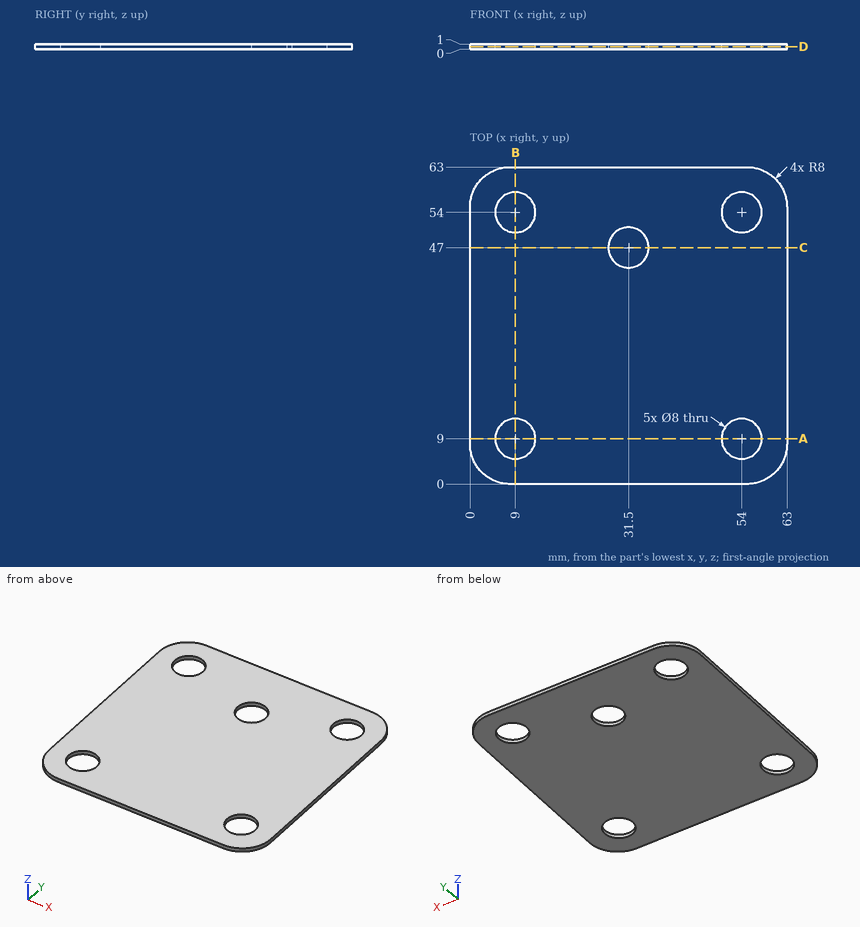
Design review of the part shown in the three views and the two pictorial views. Dimensions are in mm from the part's minimum x, y and z. Coordinates: 2 decimals unless noted, no trailing zeros. Write each loop counter-clockwise with the first axis right and the second up, starting at its lowest first coordinate (ties: lowest second). Pieces come first, ordered by that corner, then holes. Notation, with made-up numbers: (-2.5, 59.5) -> (50.5, 59.5) arc R23 ccw to (50.5, 83.5) -> close; hole circle Ø1 at (-13, 14.5). An arc over 180 degrees is marked (long way). Answer in a Markdown table with one row per item.
1. Clearance check with a flat-ended pin moving along its axis: pin 1 Ø7 at (x, y) = (54, 54) entering from -Z. State where the tip first meets the part, or that it passes through.
Answers below:
| item | result |
|---|---|
| pin 1 | passes through |
2. Wall thickness on probe 1 along Y at (x, z) = (9, 0.5); probe 2 along X at (y, z) = (10, 0.5): over which ranges is each line inside the solid? List them lowest first. Write a range as [from, to].
Answers below:
| item | result |
|---|---|
| probe 1 | y = [0, 5], [13, 50], [58, 63] |
| probe 2 | x = [0, 5.13], [12.87, 50.13], [57.87, 63] |
3. We need section A-A, the plane y = 9. State the section outline as (x, z) points, and give its area (3 significant figures).
Answers below:
| item | result |
|---|---|
| outline | (0, 0) -> (5, 0) -> (5, 1) -> (0, 1) -> close; (13, 0) -> (50, 0) -> (50, 1) -> (13, 1) -> close; (58, 0) -> (63, 0) -> (63, 1) -> (58, 1) -> close |
| area | 47.0 mm^2 |
4. We need section D-D, the plane z = 0.5. State the section outline as (x, y) points, and give its area (3 significant figures).
Answers below:
| item | result |
|---|---|
| outline | (0, 8) arc R8 ccw to (8, 0) -> (55, 0) arc R8 ccw to (63, 8) -> (63, 55) arc R8 ccw to (55, 63) -> (8, 63) arc R8 ccw to (0, 55) -> close; hole circle Ø8 at (9, 9); hole circle Ø8 at (9, 54); hole circle Ø8 at (31.5, 47); hole circle Ø8 at (54, 9); hole circle Ø8 at (54, 54) |
| area | 3,660 mm^2 |
5. We need section C-C, the plane y = 47. State the section outline as (x, z) points.
Answers below:
| item | result |
|---|---|
| outline | (0, 0) -> (27.5, 0) -> (27.5, 1) -> (0, 1) -> close; (35.5, 0) -> (63, 0) -> (63, 1) -> (35.5, 1) -> close |
